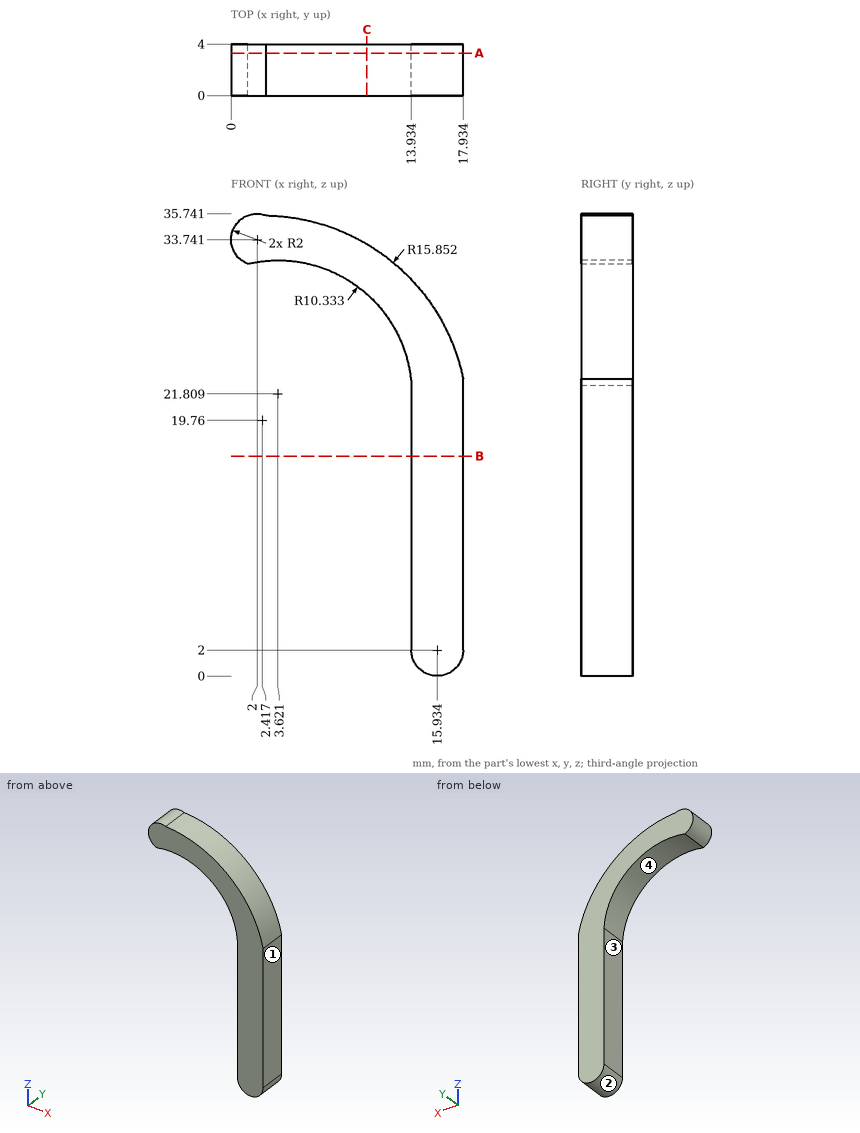
For this review, use the dimensioned drawing (mm, ordinates from the lowest corner) and the shaded views. Give positions to 0.01 mm unless a question says otherwise; leave off trailing zeros. Loops run counter-clockwise (first coordinate to the right, second up) from the corner with the lowest first, then second, coordinate; pieces in that order, holes last. Notation, with made-up numbers: (17.5, -16) -> (35.5, -16) arc R11 cw to (35.5, -12) -> close; hole circle Ø2 at (-17.75, 88). An arc over 180 degrees is marked (long way). Use CSV: the item, a comma, the result in double quotes.
1. Consider section C-C, the plane x = 10.5. Write out the cut boundary in (y, z) (1 decimal).
Result:
outline,"(0, 29.5) -> (4, 29.5) -> (4, 33.4) -> (0, 33.4) -> close"
2. To check wall thickness, follow probe 1 along X at (y, z) = (3.4, 21.5); probe 2 along X at (y, z) = (0.95, 30) (1 decimal); probe 3 along Z at (x, y) = (10.5, 2.15) (1 decimal). State the ranges of each line that lie inside material, in increasing order. Write a range as from..to.
Result:
probe 1,"x = 13.93..17.93"
probe 2,"x = 9.9..14.5"
probe 3,"z = 29.5..33.4"
3. The part is to be moulded in two halves that separate along X. For the marked faces 1, 2, 3 and 4, say which applies: +X half, -X half, draft (parallel to the pull), parting line (faces both ways), or undercut.
Result:
face 1,"+X half"
face 2,"parting line"
face 3,"-X half"
face 4,"undercut"
4. Consider section A-A, the plane y = 3.3. Write out the cut boundary in (x, z) (1 decimal), then the cut area to 3 significant figures.
Result:
outline,"(1.3, 31.9) arc R10.3 cw to (13.9, 22.5) -> (13.9, 2) arc R2 ccw to (17.9, 2) -> (17.9, 23) arc R15.9 ccw to (2.7, 35.6) arc R2 ccw to start"
area,"162 mm²"
5. For P1, Ø10, axis at x = 2.5, z = 26.5, coming from the -Y side; P2, Ø1, axis at x = 13.5, y = 2, coming from the +Z side; P3, Ø2, axis at y = 1.5, z = 9.5, coming from the -X side, all flat-tipped, find the tip position at first contact; note any pin that passes through.
Result:
P1,"passes through"
P2,"stops at z = 31.56"
P3,"stops at x = 13.93"
6. Consider section B-B, the plane z = 17. Write out the cut boundary in (x, y).
Result:
outline,"(13.93, 0) -> (17.93, 0) -> (17.93, 4) -> (13.93, 4) -> close"
